from build123d import *

# Parameters (mm, degrees)
SKETCH1_W           = 279.4
SKETCH1_H           = 279.4
SKETCH1_W_2         = 2.9972
SKETCH1_H_2         = 47.498
SKETCH1_W_3         = 40.770628572
SKETCH1_H_3         = 5.588
BOSS_EXTRUDE1_DEPTH = 1.4986
SKETCH3_R           = 1.5
CUT_EXTRUDE2_DEPTH  = 204.666583022
SKETCH4_R           = 1.5
BOSS_EXTRUDE2_DEPTH = 2.9972
SKETCH5_R           = 1.5
CUT_EXTRUDE3_DEPTH  = 216.087723417


with BuildPart() as part:
    # Sketch1 → Boss-Extrude1 (new, symmetric)
    with BuildSketch(Plane.XY):
        Rectangle(SKETCH1_W, SKETCH1_H)
        with Locations((-141.1986, -74.041)):
            Rectangle(SKETCH1_W_2, SKETCH1_H_2)
        with Locations((-81.541257143, -142.494)):
            Rectangle(SKETCH1_W_3, SKETCH1_H_3)
        with Locations((0, -142.494)):
            Rectangle(SKETCH1_W_3, SKETCH1_H_3)
        with Locations((81.541257143, -142.494)):
            Rectangle(SKETCH1_W_3, SKETCH1_H_3)
        with Locations((141.1986, -74.041)):
            Rectangle(SKETCH1_W_2, SKETCH1_H_2)
        with Locations((141.1986, 20.955)):
            Rectangle(SKETCH1_W_2, SKETCH1_H_2)
        with Locations((141.1986, 115.951)):
            Rectangle(SKETCH1_W_2, SKETCH1_H_2)
        with Locations((-141.1986, 20.955)):
            Rectangle(SKETCH1_W_2, SKETCH1_H_2)
        with Locations((-141.1986, 115.951)):
            Rectangle(SKETCH1_W_2, SKETCH1_H_2)
    extrude(amount=BOSS_EXTRUDE1_DEPTH, both=True)

    # Sketch3 → Cut-Extrude2 (cut, through all)
    with BuildSketch(Plane.XY.offset(1.4986)):
        with Locations((-128.4097, 71.374)):
            Circle(SKETCH3_R)
        with Locations((-128.4097, 55.626)):
            Circle(SKETCH3_R)
        with Locations((128.4097, 71.374)):
            Circle(SKETCH3_R)
        with Locations((128.4097, 55.626)):
            Circle(SKETCH3_R)
    extrude(amount=-CUT_EXTRUDE2_DEPTH, mode=Mode.SUBTRACT)

    # Sketch4 → Boss-Extrude2 (add)
    # profile 1 of 2: a face of its own
    with BuildSketch(Plane.XY.offset(1.4986)):
        Polygon((-142.6972, 79.4385), (-142.6972, 139.7), (-158.5722, 139.7), (-158.5722, -139.7), (-142.6972, -139.7), (-142.6972, 47.5615), (-145.3972, 47.5615), (-145.3972, 79.4385), align=None)
        with Locations((-150.6347, -133.35)):
            Circle(SKETCH4_R, mode=Mode.SUBTRACT)
    # profile 2 of 2: a face of its own
    with BuildSketch(Plane.XY.offset(1.4986)):
        Polygon((158.5722, 139.7), (142.6972, 139.7), (142.6972, 79.4385), (145.3972, 79.4385), (145.3972, 47.5615), (142.6972, 47.5615), (142.6972, -139.7), (158.5722, -139.7), align=None)
        with Locations((150.6347, -133.35)):
            Circle(SKETCH4_R, mode=Mode.SUBTRACT)
    extrude(amount=-BOSS_EXTRUDE2_DEPTH)

    # Sketch5 → Cut-Extrude3 (cut, through all)
    with BuildSketch(Plane.XY.offset(1.4986)):
        with Locations((-4.7625, 132.3975)):
            Circle(SKETCH5_R)
        with Locations((4.7625, 132.3975)):
            Circle(SKETCH5_R)
    extrude(amount=-CUT_EXTRUDE3_DEPTH, mode=Mode.SUBTRACT)


solid = part.part
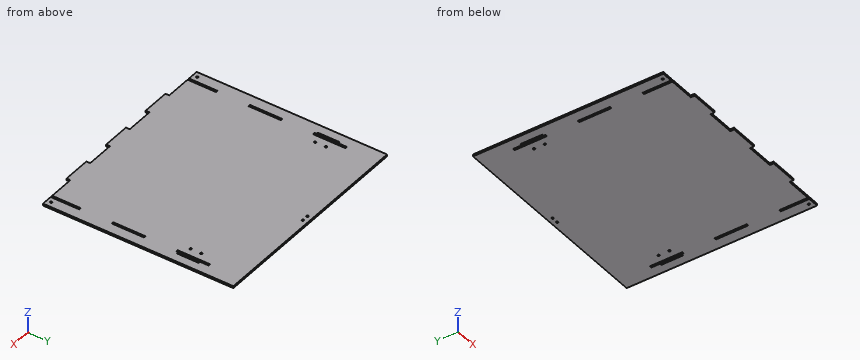
CAD build for the part. Positions are in the model's coordinates, mm. Give positions to 0.01 mm unless a question says otherwise; leave off trailing zeros. Write each loop counter-clockwise with the first axis right and the second up, starting at its lowest first coordinate (ties: lowest second). Pieces come first, ordered by that corner, then holes. Notation, with made-up numbers: (13.25, -10) - (45.25, -10) arc R3 ccw to (45.25, -6) - close; hole circle Ø6 at (-28, -33). An arc over 180 degrees is marked (long way). Answer as CSV lines item,"result".
Q1. Band-saw the part on B-B (z = 0.5). State how many separate pieces and enclosed holes the cut face has, and give its area (3 significant figures).
Result set:
separate pieces,"1"
enclosed holes,"12"
area,"88,200 mm²"
Q2. Drill centre lines: line 1 (X direction, y = 79.5, z = -0.8); line 2 (X direction, y = 78.5, z = 1.05); line 3 (Y direction, x = 128.5, z = 0.2). Where is each one in solid material? Low to high. Write a range as from..to.
Result set:
line 1,"-158.57..-142.7, -139.7..139.7, 142.7..158.57"
line 2,"-158.57..-145.4, -139.7..139.7, 145.4..158.57"
line 3,"-139.7..54.13, 57.12..69.88, 72.87..139.7"
Q3. Band-saw the part on A-A (x = 108). Give the cut face in (y, z).
Result set:
outline,"(-139.7, -1.5) - (139.7, -1.5) - (139.7, 1.5) - (-139.7, 1.5) - close"
Q4. Flat gauge pins, fed straight in: pin 1 Ø1.8 at (x, y) = (-128.41, 71.37) entering from +Z; pin 2 Ø1.5 at (y, z) = (-141, -0.5) entering from +X; pin 3 Ø1.5 at (x, z) = (147, 0) entering from -Y. Where does each tip first touch, or does it go through?
Result set:
pin 1,"through"
pin 2,"x = 101.93"
pin 3,"y = -139.7"
